Study the drawing (mm; zero at the part's minimum x, y, z) and answer. A direction names the side the tool comes from. Coordinates: 2 decimals unless noted, no trailing zeros. Order: outer loops, then holes, each group sorted by start corner. A loop starts at its lowest first (then second) coordinate and runs counter-clockwise, first axis right, second up. Notation, with made-up numbers: M -36,45 L 6,45 A30 ccw 6,77 Z; hole C -21.5,70.25 d6. An arc over 180 degrees is marked long. Put each result on its own line as item: value.
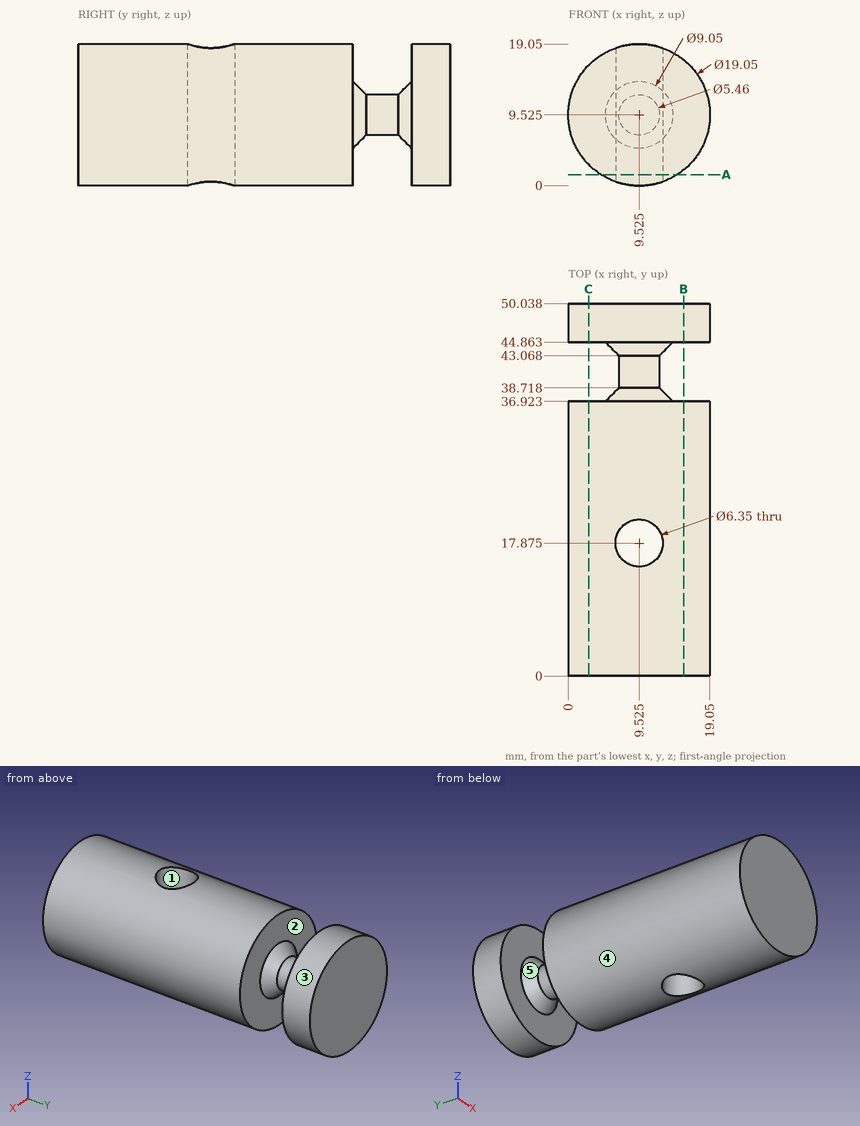
Q1. Given pin 1 (4 mm diameter, centred on x = 5, y = 29, fed in from -Z); pin 2 (3 mm diameter, centred on y = 6, z = 5, fed in from -X); pin 3 (1 mm diameter, centred on y = 35.5, z = 6.5, fed in from +X), each flat-ended and moving along its own axis, determine where each tip first touches the part or whether it passes through.
Answers below:
pin 1: stops at z = 0.34
pin 2: stops at x = 0.49
pin 3: stops at x = 18.71
Q2. For a pull along X with two mould halves and no side action, classify the marked faces 1, 2 and 3 as +X half, -X half, draft (parallel to the pull), parting line (faces both ways), or undercut.
Answers below:
face 1: undercut
face 2: draft
face 3: parting line
Q3. Consider line 1 along Y through (x, z) = (3, 4); line 2 along Y through (x, z) = (6.75, 13) (1 decimal); line 3 along Y through (x, z) = (9.5, 8.5). Determine where each line is inside the solid, lowest interval first.
Answers below:
line 1: y = 0 to 36.92, 44.86 to 50.04
line 2: y = 0 to 16.3, 19.4 to 37, 44.8 to 50
line 3: y = 0 to 14.7, 21.05 to 50.04
Q4. A tool of negligible diameter and unlimited length cuts with its end or side. For the marked faces 4 and 5, from which of +Z, -Z, +X, -X, +Y, -Y can it reach the whole face along a straight path? Write none if from no direction.
Answers below:
face 4: +Y, -Y
face 5: none
Q5. Find section A-A on z = 1.5. Give the number of separate pieces and of enclosed holes in the cut face, plus the area to 3 significant figures.
Answers below:
separate pieces: 2
enclosed holes: 1
area: 400 mm^2
Q6. Find section C-C on x = 2.75. Write down the section's boundary in (y, z).
Answers below:
outline: M 0,2.83 L 36.92,2.83 L 36.92,16.22 L 0,16.22 Z; M 44.86,2.83 L 50.04,2.83 L 50.04,16.22 L 44.86,16.22 Z
Q7. Find section B-B on x = 15.5. Write down the section's boundary in (y, z).
Answers below:
outline: M 0,2.11 L 36.92,2.11 L 36.92,16.94 L 0,16.94 Z; M 44.86,2.11 L 50.04,2.11 L 50.04,16.94 L 44.86,16.94 Z
